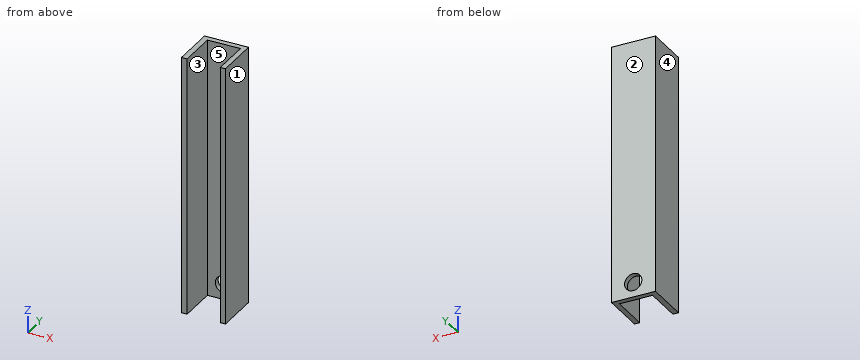
Autodesk Inventor part; units mm, degrees
ref_plane "YZ Plane" through (0, 0, 0) normal (1, 0, 0) x (0, 1, 0)
ref_plane "XZ Plane" through (0, 0, 0) normal (0, 1, 0) x (-1, 0, 0)
ref_plane "XY Plane" through (0, 0, 0) normal (0, 0, 1) x (1, 0, 0)
sketch "草圖1" plane through (0, 0, 0) normal (0, 0, 1) x (1, 0, 0)
  line L0 (0, 0) -> (0, 25.5)
  line L1 (0, 25.5) -> (25.5, 25.5)
  line L2 (25.5, 25.5) -> (25.5, 0)
  line L3 (25.5, 0) -> (0, 0)
  dimension "d0" = 25.5
  dimension "d1" = 25.5
extrude "擠出1" add sketch "草圖1" along normal blind 150
sketch "草圖2" plane through (0, 0, 150) normal (0, 0, 1) x (1, 0, 0)
  line L0 (3.28, -7.124) -> (22.5, -7.124)
  line L1 (22.5, -7.124) -> (22.5, 22.4)
  line L2 (22.5, 22.4) -> (3.28, 22.4)
  line L3 (3.28, 22.4) -> (3.28, -7.124)
  line L4 (0, 0) -> (25.5, 0)
  dimension "d4" = 19.22
  dimension "d5" = 22.4
  dimension "d6" = 3
extrude "擠出2" cut sketch "草圖2" against normal through all
sketch "草圖3" plane through (3.28, 22.4, 150) normal (0, -1, 0) x (1, 0, 0)
  circle A0 centre (9.61, -141.2584) radius 5
  point P0 (-3.28, -150)
  dimension "d9" = 10
extrude "擠出3" cut sketch "草圖3" against normal blind 150
properties part number "ㄇ形件" material "鋁合金 6061"
Input: part model. Units: mm. Frame: model coordinates. Face numbers are marked on the shaded views. A direction names the side the tool comes from. Give positions to 0.01 mm unless a question says otherwise; leave off trailing zeros. Loops run counter-clockwise (first coordinate to the right, second up) from the corner with the lowest first, then second, coordinate; pieces in that order, holes last. Notation, with made-up numbers: M 45.5,37 L 82.5,37 A7 ccw 82.5,46 Z; hole C 56,34 d4. An arc over 180 degrees is marked long. Use one line per item in the form item = value.
1. Pull-direction query (X, two-part tool) for the marked faces 1, 2 and 3; classes: released by +X, released by -X, zero draft, split by the parting line, or undercut.
Numbers:
face_1 = released by +X
face_2 = zero draft
face_3 = undercut
2. Reachability of the marked faces 4 and 5 from +Z, -Z, +X, -X, +Y, -Y: full face, straight path, thin tool, end or side. Return the list, or none.
Numbers:
face_4 = +Z, -Z, -X, +Y, -Y
face_5 = +Z, -Z, -Y
3. Section query C-C, the plane z = 29. Return the cut outline in (x, y), and give its area (3 significant figures).
Numbers:
outline = M 0,0 L 3.28,0 L 3.28,22.4 L 22.5,22.4 L 22.5,0 L 25.5,0 L 25.5,25.5 L 0,25.5 Z
area = 220 mm²
4. Section query A-A, the plane x = 12.89. Return the cut outline in (y, z), and give its area (3 significant figures).
Numbers:
outline = M 22.4,0 L 25.5,0 L 25.5,3.74 L 22.4,3.74 Z; M 22.4,13.74 L 25.5,13.74 L 25.5,150 L 22.4,150 Z
area = 434 mm²
5. First-contact query: pin 1 (2 mm diameter, centred on x = 20, z = 20, fed in from -Y). Flat tip, straight axial feed; report the tip coordinate or a pass-through.
Numbers:
pin_1 = 22.4
6. Section query D-D, the plane x = 21. Return the cut outline in (y, z).
Numbers:
outline = M 22.4,0 L 25.5,0 L 25.5,150 L 22.4,150 Z
7. Line query: L1, parallel to X at y = 9, z = 44; L2, parallel to Z at x = 12.89, y = 24.75; L3, parallel to Y at x = 18, z = 95.5. Output: solid intervals per line, ascending.
Numbers:
L1 = 0 to 3.28, 22.5 to 25.5
L2 = 0 to 3.74, 13.74 to 150
L3 = 22.4 to 25.5
8. Section query B-B, the plane y = 15.25. Return the cut outline in (x, z), and give its area (3 significant figures).
Numbers:
outline = M 0,0 L 3.28,0 L 3.28,150 L 0,150 Z; M 22.5,0 L 25.5,0 L 25.5,150 L 22.5,150 Z
area = 942 mm²
